from build123d import *

# Parameters (mm, degrees)
BOSS_EXTRUDE1_DEPTH = 8.5
SKETCH2_R           = 9
CUT_EXTRUDE1_DEPTH  = 117.679046962


with BuildPart() as part:
    # Sketch1 → Boss-Extrude1 (new, symmetric)
    with BuildSketch(Plane.XY):
        with BuildLine():
            Line((0, 110), (35, 110))
            Line((35, 110), (35, 87))
            ThreePointArc((35, 87), (22.888974491, 47), (35, 7))
            Line((35, 7), (35, 0))
            Line((35, 0), (0, 0))
            Line((0, 0), (0, 110))
        make_face()
    extrude(amount=BOSS_EXTRUDE1_DEPTH, both=True)

    # Sketch2 → Cut-Extrude1 (cut, through all)
    with BuildSketch(Plane.XY.offset(8.5)):
        with Locations((18, 92)):
            Circle(SKETCH2_R)
        with Locations((18, 17)):
            Circle(SKETCH2_R)
    extrude(amount=-CUT_EXTRUDE1_DEPTH, mode=Mode.SUBTRACT)


solid = part.part
Could you check a few things on this model? Use its own coordinates, in mm. Coordinates: 2 decimals unless noted, no trailing zeros. Write each loop counter-clockwise with the first axis right and the second up, starting at its lowest first coordinate (ties: lowest second). Pieces come first, ordered by that corner, then holes. Notation, with made-up numbers: M -23,38 L -9,38 A34 ccw -9,72 Z; hole C -20,48 d4. An arc over 180 degrees is marked long. One line per question, with ' | ' between items.
1) Imagine slicing it at A-A, the plane x = 18. Write out the boundary of the cut face in (y, z).
Checks:
outline: M 0,-8.5 L 8,-8.5 L 8,8.5 L 0,8.5 Z; M 26,-8.5 L 83,-8.5 L 83,8.5 L 26,8.5 Z; M 101,-8.5 L 110,-8.5 L 110,8.5 L 101,8.5 Z
2) Imagine slicing it at C-C, the plane z = 5.5. Write out the boundary of the cut face in (x, y), and give its area (3 significant figures).
Checks:
outline: M 0,0 L 35,0 L 35,7 A72.11 cw 35,87 L 35,110 L 0,110 Z; hole C 18,17 d18; hole C 18,92 d18 | area: 2,680 mm²
3) I need wall thicknesses on probe 1 along Y at (x, z) = (18, -2.5); probe 2 along Y at (x, z) = (22, 6); probe 3 along X at (y, z) = (22.5, 3.75). Which ranges of each line are inside material? Lowest first, please. Write a range as [from, to].
Checks:
probe 1: [0, 8], [26, 83], [101, 110] | probe 2: [0, 8.94], [25.06, 83.94], [100.06, 110] | probe 3: [0, 10.88], [25.12, 27.18]
4) Imagine slicing it at D-D, the plane x = 30. Write out the boundary of the cut face in (y, z), and give its area (3 significant figures).
Checks:
outline: M 0,-8.5 L 15.78,-8.5 L 15.78,8.5 L 0,8.5 Z; M 78.22,-8.5 L 110,-8.5 L 110,8.5 L 78.22,8.5 Z | area: 808 mm²
5) If we mould it in two halves opening along Y, with no side actions, what happens to faces 1 (the face through (22.153, 84.015, 0.119)), 2 (the face through (22.89, 47.59, 0.12)), 3 (the face through (14, 56, -8.5)), 4 (the face through (18, 0, 0))? For each: released by +Y, released by -Y, zero draft, split by the parting line, or undercut.
Checks:
face 1: undercut | face 2: undercut | face 3: zero draft | face 4: released by -Y
6) Imagine slicing it at B-B, the plane y = 92. Write out the boundary of the cut face in (x, z).
Checks:
outline: M 0,-8.5 L 9,-8.5 L 9,8.5 L 0,8.5 Z; M 27,-8.5 L 35,-8.5 L 35,8.5 L 27,8.5 Z
7) For pin 1 Ø1.5 at (y, z) = (56, -3.5) entering from +X; pin 2 Ø16 at (x, y) = (18, 92) entering from -Z; pin 3 Ø2 at (y, z) = (66.5, 1) entering from +X, each with a flat end and sliding along its axis, tell me the tip position at first contact or that it passes through.
Checks:
pin 1: x = 23.55 | pin 2: through | pin 3: x = 25.86
